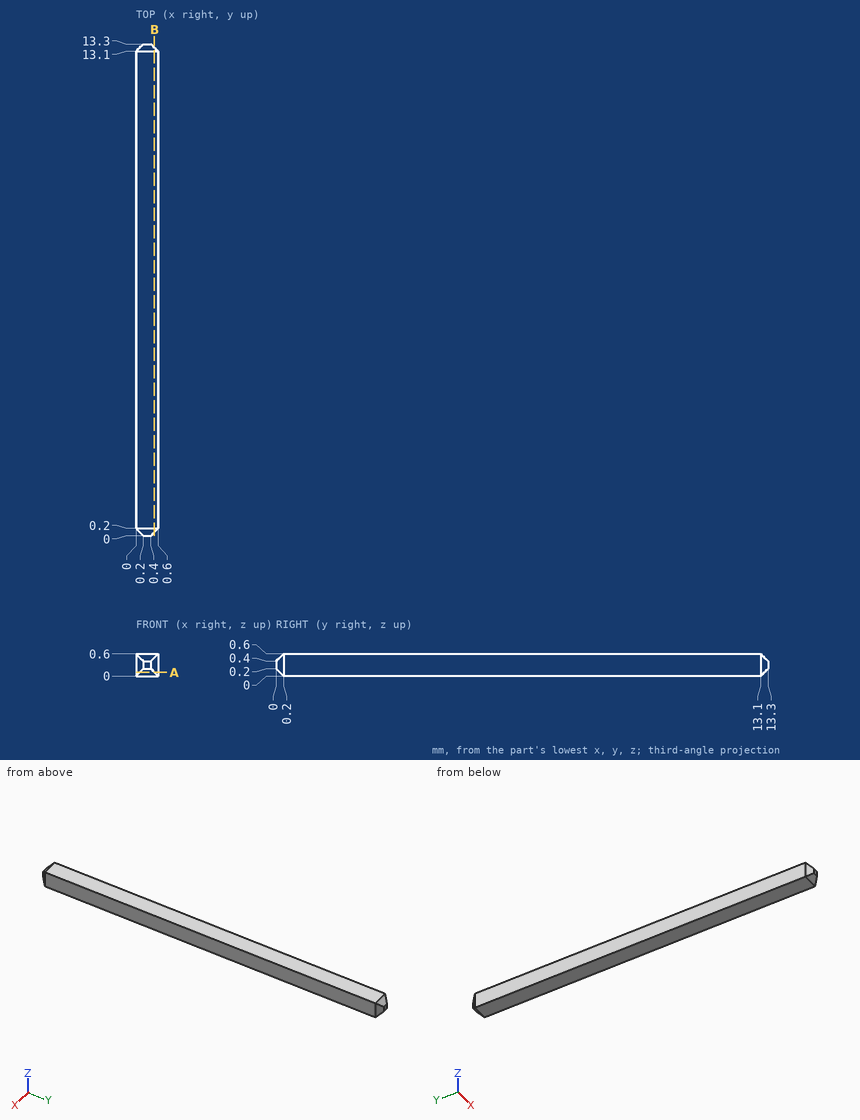
The figure shows three views and two pictorial views of one solid part (mm, origin at its lowest corner). Answer the questions. Coordinates: 2 decimals unless noted, no trailing zeros. Order: outer loops, then holes, each group sorted by start corner. A loop starts at its lowest first (then second) coordinate and runs counter-clockwise, first axis right, second up.
Q1. A cutting plane is placed at A-A, the plane z = 0.1. Write down the section's boundary in (x, y), and give its area (3 significant figures).
Q2. A cutting plane is placed at B-B, the plane x = 0.5. Write down the section's boundary in (y, z).
Q3. Consider line 1 (Y direction, x = 0.5, z = 0.35); line 2 (Y direction, x = 0.2, z = 0.15). Determine where each line is inside the solid, lowest interval first.
Answers follow:
1. outline: (0, 0.2) - (0.1, 0.1) - (0.5, 0.1) - (0.6, 0.2) - (0.6, 13.1) - (0.5, 13.2) - (0.1, 13.2) - (0, 13.1) - close
1. area: 7.84 mm2
2. outline: (0.1, 0.1) - (0.2, 0) - (13.1, 0) - (13.2, 0.1) - (13.2, 0.5) - (13.1, 0.6) - (0.2, 0.6) - (0.1, 0.5) - close
3. line 1: y = 0.1 to 13.2
3. line 2: y = 0.05 to 13.25
